Check sheet for the drawn part. Datum: minimum x, y, z corner. Units: mm. A direction names the side the tool comes from. Round coordinates to 2 decimals unless told otherwise and drop trailing zeros. Loops run counter-clockwise (first coordinate to the right, second up) from the corner with the lowest first, then second, coordinate; pieces in that order, holes last. Notation, with made-up numbers: (1, 32) -> (53, 32) arc R17 ccw to (53, 46) -> close; hole circle Ø10 at (3.5, -14.5). An arc over 180 degrees is marked (long way). Return JSON: item names as keys, results as strings.
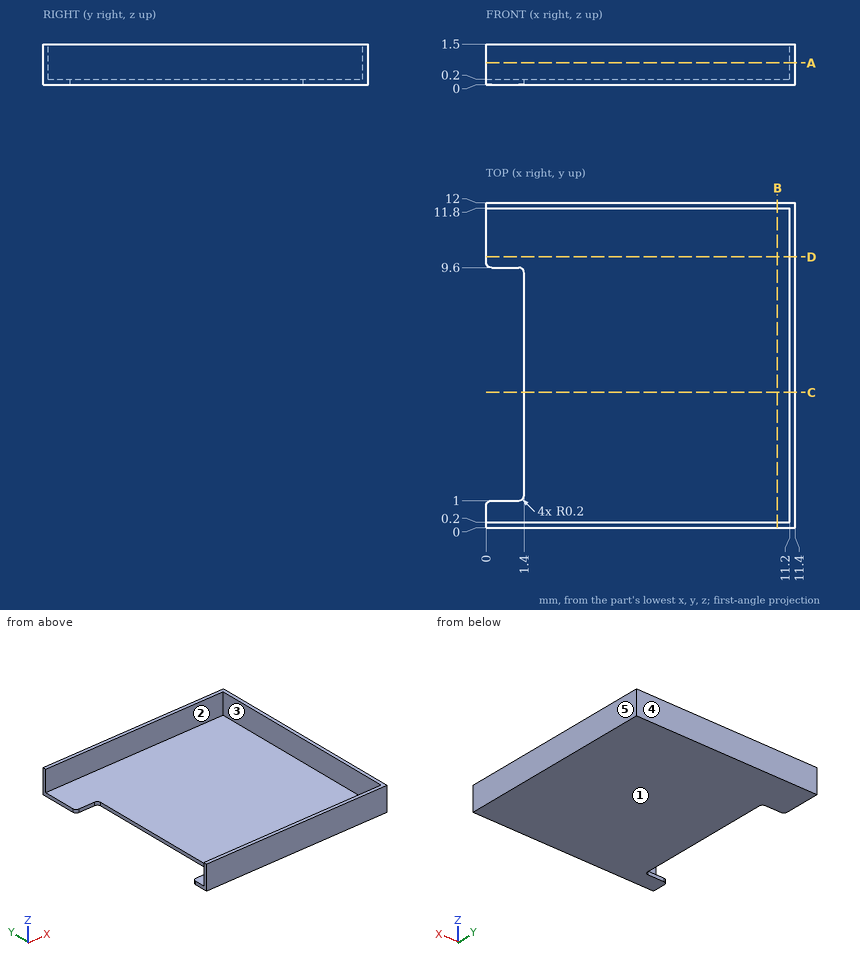
Q1. Section check A-A (z = 0.8). Record the boundary of the cut face in (x, y), then the cut area to 3 significant figures.
Results list:
{"outline": "(0, 0) -> (11.4, 0) -> (11.4, 12) -> (0, 12) -> (0, 11.8) -> (11.2, 11.8) -> (11.2, 0.2) -> (0, 0.2) -> close", "area": "6.88 mm^2"}
Q2. Go/stop test with flat-tipped pins: pin 1 (3 mm diameter, centred on x = 6.5, y = 7, fed in from +Z); pin 2 (0.7 mm diameter, centred on y = 8.5, z = 0.5, fed in from -X). Record where each tip stops, or that it passes through.
Results list:
{"pin 1": "z = 0.2", "pin 2": "x = 1.4"}
Q3. Draft check along Y on the marked faces 3, 4 and 5. Enter one of: released by +Y, released by -Y, zero draft, split by the parting line, or undercut.
Results list:
{"face 3": "undercut", "face 4": "released by +Y", "face 5": "zero draft"}
Q4. Material ranges on line 1 (Y direction, x = 9.5, z = 0.65); line 2 (X direction, y = 3.75, z = 0.7); line 3 (Z direction, x = 7, y = 6.5), recorded low to high.
Results list:
{"line 1": "0 to 0.2, 11.8 to 12", "line 2": "11.2 to 11.4", "line 3": "0 to 0.2"}
Q5. Section check D-D (y = 10). Record the boundary of the cut face in (x, z).
Results list:
{"outline": "(0, 0) -> (11.4, 0) -> (11.4, 1.5) -> (11.2, 1.5) -> (11.2, 0.2) -> (0, 0.2) -> close"}
Q6. Tool access check on the marked faces 1 and 2. Record the directions out of +Z, -Z, +X, -X, +Y, -Y that give a thin tool (end or side, any length) a straight path to the whole face; none if there is none.
Results list:
{"face 1": "-Z, +X, -X, +Y, -Y", "face 2": "+Z, -X"}
Q7. Section check C-C (y = 5). Record the boundary of the cut face in (x, z).
Results list:
{"outline": "(1.4, 0) -> (11.4, 0) -> (11.4, 1.5) -> (11.2, 1.5) -> (11.2, 0.2) -> (1.4, 0.2) -> close"}
Q8. Section check B-B (x = 10.75). Record the boundary of the cut face in (y, z).
Results list:
{"outline": "(0, 0) -> (12, 0) -> (12, 1.5) -> (11.8, 1.5) -> (11.8, 0.2) -> (0.2, 0.2) -> (0.2, 1.5) -> (0, 1.5) -> close"}
